from build123d import *

# Parameters (mm, degrees)
SKETCH_1_R          = 2.2
SKETCH_1_R_2        = 2.7
EXTRUDE_1_DEPTH     = 5
CUT_EXTRUDE_1_REACH = 59.23
EXTRUDE_START       = -5
SKETCH_6_W          = 7
SKETCH_6_H          = 3
SKETCH_6_R          = 2.7
EXTRUDE_3_DEPTH     = 5
CUT_EXTRUDE_2_REACH = 45.949
SKETCH_8_R          = 1
FILLET_1_R          = 2


with BuildPart() as part:
    # 草图1 → 凸台-拉伸1 (new body)
    with BuildSketch(Plane.XY):
        with BuildLine():
            Line((-21.928513003, 31.619793089), (-45, 12.5))
            Line((-45, 12.5), (-45, -12.5))
            Line((-45, -12.5), (-21.928513003, -31.619793089))
            ThreePointArc((-21.928513003, -31.619793089), (-18.386291168, -32.993165888), (-14.729286549, -31.963697294))
            Line((-14.729286549, -31.963697294), (22.594284602, -6.618263059))
            ThreePointArc((22.594284602, -6.618263059), (26.1, 0), (22.594284602, 6.618263059))
            Line((22.594284602, 6.618263059), (-14.729286549, 31.963697294))
            ThreePointArc((-14.729286549, 31.963697294), (-18.386291168, 32.993165888), (-21.928513003, 31.619793089))
        make_face()
        with Locations((-18.1, -8)):
            Circle(SKETCH_1_R, mode=Mode.SUBTRACT)
        with Locations((-18.1, 8)):
            Circle(SKETCH_1_R, mode=Mode.SUBTRACT)
        with Locations((-34.1, 0)):
            Circle(SKETCH_1_R, mode=Mode.SUBTRACT)
        with Locations((-18.1, 27)):
            Circle(SKETCH_1_R_2, mode=Mode.SUBTRACT)
        with Locations((-18.1, -27)):
            Circle(SKETCH_1_R_2, mode=Mode.SUBTRACT)
        with Locations((18.1, 0)):
            Circle(SKETCH_1_R_2, mode=Mode.SUBTRACT)
    extrude(amount=EXTRUDE_1_DEPTH)

    # 草图4 → 旋转1 (revolve)
    with BuildSketch(Plane(origin=(-24.93598604, 16.933358057, 0), x_dir=(0, 0, -1), z_dir=(0.8272828823621655, -0.5617855752425007, 0)), mode=Mode.PRIVATE) as revolve_1_sk:
        Polygon((7.7, 17.168318912), (7.7, 14.868318912), (0, 14.868318912), (0, 18.168318912), align=None)
    revolve_1 = revolve(revolve_1_sk.sketch.rotate(Axis((-18.1, 27, 1000.278995542), (0, 0, -1)), 55.820627671), axis=Axis((-18.1, 27, 1000.278995542), (0, 0, -1)))

    # 镜向1: 旋转1 across plane
    add(revolve_1.mirror(Plane.ZX))

    # 草图5 → 切除-拉伸1 (cut, up to next)
    with BuildSketch(Plane.XY.offset(5), mode=Mode.PRIVATE) as cut_extrude_1_sk1:
        with BuildLine():
            Line((-24.1, -27), (-24.1, 27))
            ThreePointArc((-24.1, 27), (-23.53005884, 29.552344215), (-21.928513003, 31.619793089))
            Line((-21.928513003, 31.619793089), (-45, 12.5))
            Line((-45, 12.5), (-45, -12.5))
            Line((-45, -12.5), (-21.928513003, -31.619793089))
            ThreePointArc((-21.928513003, -31.619793089), (-23.53005884, -29.552344215), (-24.1, -27))
        make_face()
    cut_extrude_1_tool1 = extrude(cut_extrude_1_sk1.sketch, amount=-CUT_EXTRUDE_1_REACH, mode=Mode.PRIVATE) & part.part
    add(cut_extrude_1_tool1.solids().sort_by_distance((-33.100815, 0, 5))[0], mode=Mode.SUBTRACT)

    # 草图6 → 凸台-拉伸3 (add)
    with BuildSketch(Plane.XY.offset(5).offset(EXTRUDE_START)):
        Polygon((12.5, -13.473020485), (-14.729286549, -31.963697294), (12.5, -31.963697294), (12.5, -21), (23.5, -21), (23.5, 21), (12.5, 21), (12.5, 31.963697294), (-14.729286549, 31.963697294), (12.5, 13.473020485), align=None)
        with Locations((18, -16)):
            Rectangle(SKETCH_6_W, SKETCH_6_H, mode=Mode.SUBTRACT)
        with Locations((18.1, 0)):
            Circle(SKETCH_6_R, mode=Mode.SUBTRACT)
        with Locations((18, 16)):
            Rectangle(SKETCH_6_W, SKETCH_6_H, mode=Mode.SUBTRACT)
    extrude(amount=EXTRUDE_3_DEPTH)

    # 草图8 → 切除-拉伸2 (cut, up to next)
    with BuildSketch(Plane.XY.offset(5), mode=Mode.PRIVATE) as cut_extrude_2_sk1:
        with Locations((9.5, -26.963697294)):
            Circle(SKETCH_8_R)
    cut_extrude_2_tool1 = extrude(cut_extrude_2_sk1.sketch, amount=-CUT_EXTRUDE_2_REACH, mode=Mode.PRIVATE) & part.part
    # 草图8 → 切除-拉伸2 (cut, up to next)
    with BuildSketch(Plane.XY.offset(5), mode=Mode.PRIVATE) as cut_extrude_2_sk2:
        with Locations((3, -26.963697294)):
            Circle(SKETCH_8_R)
    cut_extrude_2_tool2 = extrude(cut_extrude_2_sk2.sketch, amount=-CUT_EXTRUDE_2_REACH, mode=Mode.PRIVATE) & part.part
    # 草图8 → 切除-拉伸2 (cut, up to next)
    with BuildSketch(Plane.XY.offset(5), mode=Mode.PRIVATE) as cut_extrude_2_sk3:
        with Locations((9.5, 26.963697294)):
            Circle(SKETCH_8_R)
    cut_extrude_2_tool3 = extrude(cut_extrude_2_sk3.sketch, amount=-CUT_EXTRUDE_2_REACH, mode=Mode.PRIVATE) & part.part
    # 草图8 → 切除-拉伸2 (cut, up to next)
    with BuildSketch(Plane.XY.offset(5), mode=Mode.PRIVATE) as cut_extrude_2_sk4:
        with Locations((3, 26.963697294)):
            Circle(SKETCH_8_R)
    cut_extrude_2_tool4 = extrude(cut_extrude_2_sk4.sketch, amount=-CUT_EXTRUDE_2_REACH, mode=Mode.PRIVATE) & part.part
    add(cut_extrude_2_tool1.solids().sort_by_distance((9.5, -26.963697, 5))[0], mode=Mode.SUBTRACT)
    add(cut_extrude_2_tool2.solids().sort_by_distance((3, -26.963697, 5))[0], mode=Mode.SUBTRACT)
    add(cut_extrude_2_tool3.solids().sort_by_distance((9.5, 26.963697, 5))[0], mode=Mode.SUBTRACT)
    add(cut_extrude_2_tool4.solids().sort_by_distance((3, 26.963697, 5))[0], mode=Mode.SUBTRACT)

    # 草图7 → 旋转2 (revolve)
    with BuildSketch(Plane(origin=(6.469864276, 8.674410623, 0), x_dir=(0.8015915013283047, -0.5978721142503927, 0), z_dir=(0.5978721142503927, 0.8015915013283047, 0)), mode=Mode.PRIVATE) as revolve_2_sk:
        Polygon((11.808806174, 7.7), (11.808806174, 0), (8.508806174, 0), (9.508806174, 7.7), align=None)
    revolve(revolve_2_sk.sketch.rotate(Axis((18.1, 0, 1), (0, 0, -1)), 143.282349417), axis=Axis((18.1, 0, 1), (0, 0, -1)))

    # 圆角1
    fillet_1_edges = [part.edges().sort_by_distance(p)[0] for p in [
        (12.5, 31.963697294, 2.5),
        (12.5, 21, 2.5),
        (23.5, 21, 2.5),
        (12.5, -21, 2.5),
        (23.5, -21, 2.5),
        (12.5, -31.963697294, 2.5),
    ]]
    fillet(fillet_1_edges, radius=FILLET_1_R)


solid = part.part
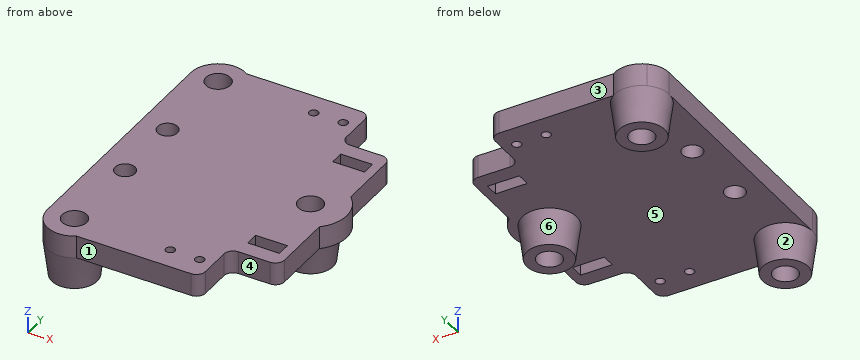
Check sheet for the modelled part. Datum: model origin and axes. Units: mm. Face numbers are marked on the shaded views. A direction names the side the tool comes from. Coordinates: 2 decimals unless noted, no trailing zeros. Write each loop counter-clockwise with the first axis right and the second up, starting at its lowest first coordinate (ties: lowest second). Pieces come first, ordered by that corner, then holes.
Item 1: Scan lines: probe 1 along Y at (x, z) = (-18.1, 2); probe 2 along Y at (x, z) = (3, 2.9); probe 3 along Y at (x, z) = (18.1, 1.6). Record each from-to range of solid material in increasing order.
Numbers:
probe 1: y = -33 to -29.7, -24.3 to -10.2, -5.8 to 5.8, 10.2 to 24.3, 29.7 to 33
probe 2: y = -31.96 to -27.96, -25.96 to 25.96, 27.96 to 31.96
probe 3: y = -21 to -17.5, -14.5 to -2.7, 2.7 to 14.5, 17.5 to 21
Item 2: Cross-section at A-A on x = 18.1. Record the boundary of the cut face in (y, z), then the cut area to 3 significant figures.
Numbers:
outline: (-21, 0) - (-17.5, 0) - (-17.5, 5) - (-21, 5) - close; (-14.5, 0) - (-6, 0) - (-5, -7.7) - (-2.7, -7.7) - (-2.7, 5) - (-14.5, 5) - close; (2.7, -7.7) - (5, -7.7) - (6, 0) - (14.5, 0) - (14.5, 5) - (2.7, 5) - close; (17.5, 0) - (21, 0) - (21, 5) - (17.5, 5) - close
area: 196 mm2
Item 3: Cross-section at B-B on x = -18.1. Record the boundary of the cut face in (y, z), then the cut area to 3 significant figures.
Numbers:
outline: (-33, 0) - (-32, -7.7) - (-29.7, -7.7) - (-29.7, 5) - (-33, 5) - close; (-24.3, -7.7) - (-22, -7.7) - (-21, 0) - (-10.2, 0) - (-10.2, 5) - (-24.3, 5) - close; (-5.8, 0) - (5.8, 0) - (5.8, 5) - (-5.8, 5) - close; (10.2, 0) - (21, 0) - (22, -7.7) - (24.3, -7.7) - (24.3, 5) - (10.2, 5) - close; (29.7, -7.7) - (32, -7.7) - (33, 0) - (33, 5) - (29.7, 5) - close
area: 318 mm2
Item 4: Cross-section at D-D on y = -8. Record the boundary of the cut face in (x, z).
Numbers:
outline: (-24.1, 0) - (-20.3, 0) - (-20.3, 5) - (-24.1, 5) - close; (-15.9, 0) - (23.5, 0) - (23.5, 5) - (-15.9, 5) - close
Item 5: Cross-section at C-C on z = -1.25. Record the boundary of the cut face in (x, y), then the cut area to 3 significant figures.
Numbers:
outline: circle Ø11.68 at (-18.1, -27); circle Ø11.68 at (-18.1, 27); circle Ø11.68 at (18.1, 0); hole circle Ø5.4 at (-18.1, -27); hole circle Ø5.4 at (-18.1, 27); hole circle Ø5.4 at (18.1, 0)
area: 252 mm2
Item 6: Mould release check, pull along Y, two halves, no side actions. Record for the marked faces 4, 5 and 6: released by +Y, released by -Y, zero draft, split by the parting line, or undercut.
Numbers:
face 4: released by -Y
face 5: undercut
face 6: split by the parting line
Item 7: Depth check by flat-ended pin: pin 1 Ø4 at (y, z) = (-12.5, 2) entering from +X; pin 2 Ø5.5 at (x, z) = (-3, 1.5) entering from -Y; pin 3 Ø3 at (x, y) = (-17, 7) entering from +Z; pin 4 Ø4 at (x, z) = (18.5, -4) entering from +Y. Enter the tip coordinate at first touch or a pass-through.
Numbers:
pin 1: stops at x = 23.5
pin 2: stops at y = -31.96
pin 3: stops at z = 5
pin 4: stops at y = 5.74
Item 8: Access from +Z, -Z, +X, -X, +Y, -Y to the whole of each face (thin tool, end or side, straight path). Record for the marked faces 1, 2 and 3.
Numbers:
face 1: +Z, -Z, +X, -Y
face 2: -Z
face 3: +Z, -Z, +X, +Y
